The listing builds one solid part. Answer for the finished solid, in the listing's coordinates (mm). A direction names the side the tool comes from. Coordinates: 2 decimals unless noted, no trailing zeros. Loops run counter-clockwise (first coordinate to the right, second up) from the corner with the lowest first, then second, coordinate; pieces in that order, holes last. Notation, with made-up numbers: (-31, 59.25) - (-3, 59.25) arc R11 cw to (-3, 72.25) - close; hole circle Ø10 at (0.5, 87.5). An arc over 180 degrees is marked (long way). Return JSON: item names as keys, results as strings. Group by question number.
1. Section C-C (z = 12.75) is taken. Write down the section's boundary in (x, y), and give its area (3 significant figures).
2. The mould has two halves that part along X. Classify faces 6 (the face through (-8.25, -0.1, 14.5)), 7 (the face through (5.25, 0, 8)), 8 (the face through (-0.1, -8.25, 14.5)): pulls with the +X half, pulls with the -X half, needs draft (parallel to the pull), parting line crosses it, or undercut.
3. Section D-D (x = 5.5) is taken. Write down the section's boundary in (y, z), and give its area (4 significant figures).
4. Each of these flat-tipped pins is pushed along its axis until it touches: P1, Ø3, axis at y = 1.5, z = 9.5, coming from the +X side; P2, Ø4, axis at x = -5, y = -2.5, coming from the +Z side; P3, Ø6, axis at y = 5, z = 2.5, coming from the -X side; P4, Ø2, axis at x = 5.5, z = 9, coming from the +Y side. Where does it stop, or does it pass through?
5. Which of the six approach directions +Z, -Z, +X, -X, +Y, -Y give full straight-line access (tool end or side, diameter ignored) to faces 1 (the face through (0, -5.25, 8)), 2 (the face through (0, 6.25, 7)), 3 (the face through (-6.25, 0, 7)), 4 (the face through (6.25, 0, 7)), 5 (the face through (0, -6.25, 7))?
6. Section A-A (x = 3.25) is taken. Write down the section's boundary in (y, z), and give its area (3 significant figures).
7. Find the intervals of material crossed by line 1 along X through (y, z) = (-1, 8.25); line 2 along Z through (x, y) = (-6.25, -6.5), in increasing order.
```python
from build123d import *

# Parameters (mm, degrees)
SKETCH1_W           = 12.5
SKETCH1_H           = 12.5
BOSS_EXTRUDE1_DEPTH = 15
SHELL3_T            = -1
SKETCH2_W           = 16.5
SKETCH2_H           = 16.5
SKETCH2_W_2         = 12.5
SKETCH2_H_2         = 12.5
BOSS_EXTRUDE2_DEPTH = 1


with BuildPart() as part:
    # Sketch1 → Boss-Extrude1 (new body)
    with BuildSketch(Plane.XY):
        Rectangle(SKETCH1_W, SKETCH1_H)
    extrude(amount=BOSS_EXTRUDE1_DEPTH)

    # Shell3
    shell3_openings = [part.faces().sort_by_distance(p)[0] for p in [
        (0, 0, 15),
    ]]
    offset(amount=SHELL3_T, openings=shell3_openings, kind=Kind.INTERSECTION)

    # Sketch2 → Boss-Extrude2 (add)
    with BuildSketch(Plane.XY.offset(15)):
        Rectangle(SKETCH2_W, SKETCH2_H)
        Rectangle(SKETCH2_W_2, SKETCH2_H_2, mode=Mode.SUBTRACT)
    extrude(amount=-BOSS_EXTRUDE2_DEPTH)


solid = part.part
```
The answers:
{
 "1": {"outline": "(-6.25, -6.25) - (6.25, -6.25) - (6.25, 6.25) - (-6.25, 6.25) - close; hole (-5.25, -5.25) - (5.25, -5.25) - (5.25, 5.25) - (-5.25, 5.25) - close", "area": "46.0 mm2"},
 "2": {"face 6": "pulls with the -X half", "face 7": "undercut", "face 8": "needs draft"},
 "3": {"outline": "(-8.25, 14) - (-6.25, 14) - (-6.25, 0) - (6.25, 0) - (6.25, 14) - (8.25, 14) - (8.25, 15) - (-8.25, 15) - close", "area": "191.5 mm2"},
 "4": {"P1": "stops at x = 6.25", "P2": "stops at z = 15", "P3": "stops at x = -6.25", "P4": "stops at y = 6.25"},
 "5": {"face 1": "+Z", "face 2": "-Z, +X, -X, +Y", "face 3": "-Z, -X, +Y, -Y", "face 4": "-Z, +X, +Y, -Y", "face 5": "-Z, +X, -X, -Y"},
 "6": {"outline": "(-8.25, 14) - (-6.25, 14) - (-6.25, 0) - (6.25, 0) - (6.25, 14) - (8.25, 14) - (8.25, 15) - (5.25, 15) - (5.25, 1) - (-5.25, 1) - (-5.25, 15) - (-8.25, 15) - close", "area": "44.5 mm2"},
 "7": {"line 1": "x = -6.25 to -5.25, 5.25 to 6.25", "line 2": "z = 14 to 15"}
}
